Input: dimensioned drawing with shaded views. Units: mm. Origin: part minimum x, y, z. Give positions to 0.01 mm unless a question says otherwise; leave off trailing zeros. Order: outer loops, then holes, each group sorted by start corner. A loop starts at its lowest first (then second) coordinate and runs counter-clockwise, first axis right, second up. Notation, with made-up numbers: M -25,13.25 L 6,13.25 A18 cw 6,29.25 Z; hole C 34,22.25 d6. An arc over 180 degrees is marked long. Answer in a Markdown table with one row per item. Add a question column.
(1) Section query A-A, the plane x = 15. Return loops of the section in (y, z).
(2) Section query C-C, the plane y = 7. Return loops of the section in (x, z), plus the area to 3 significant figures.
(3) Material intervals for line 1 along Y through (x, z) = (28, 6); line 2 along Y through (x, z) = (32, 9.25); line 3 along X through (y, z) = (6.5, 8.75) (1 decimal), sorted ascending.
(4) Section query D-D, the plane y = 11. Return loops of the section in (x, z).
(5) Section query B-B, the plane z = 4. Return loops of the section in (x, y).
(6) Pin query (flat end, axial travel): P1, Ø1.5, axis at y = 10, z = 3.5, coming from the +X side; P2, Ø6, axis at x = 54, z = 1, coming from the -Y side. Return the tip coordinate at first contact, or that it passes through.
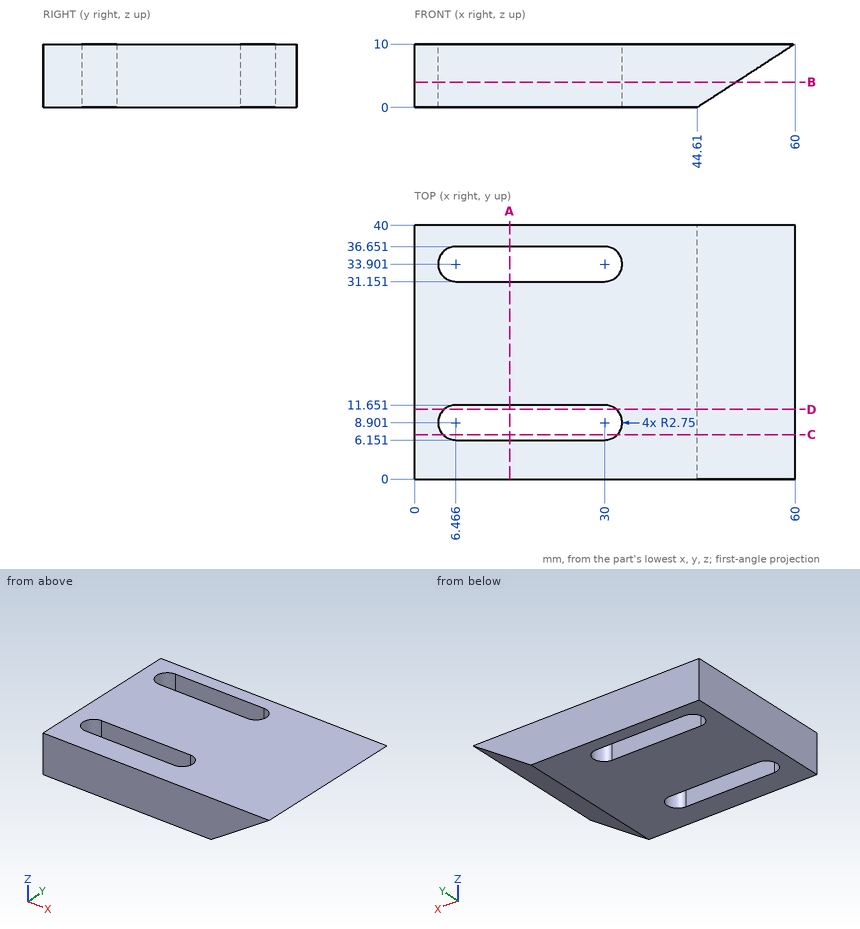
Values follow:
| question | item | result |
|---|---|---|
| 1 | outline | M 0,0 L 6.15,0 L 6.15,10 L 0,10 Z; M 11.65,0 L 31.15,0 L 31.15,10 L 11.65,10 Z; M 36.65,0 L 40,0 L 40,10 L 36.65,10 Z |
| 2 | outline | M 0,0 L 4.48,0 L 4.48,10 L 0,10 Z; M 31.99,0 L 44.61,0 L 60,10 L 31.99,10 Z |
| 2 | area | 248 mm² |
| 3 | line 1 | y = 0 to 6.15, 11.65 to 31.15, 36.65 to 40 |
| 3 | line 2 | y = 0 to 7.01, 10.79 to 32.01, 35.79 to 40 |
| 3 | line 3 | x = 0 to 5.1, 31.3 to 58.1 |
| 4 | outline | M 0,0 L 4.69,0 L 4.69,10 L 0,10 Z; M 31.78,0 L 44.61,0 L 60,10 L 31.78,10 Z |
| 5 | outline | M 0,0 L 50.77,0 L 50.77,40 L 0,40 Z; hole M 6.47,6.15 L 30,6.15 A2.75 ccw 30,11.65 L 6.47,11.65 A2.75 ccw Z; hole M 6.47,31.15 L 30,31.15 A2.75 ccw 30,36.65 L 6.47,36.65 A2.75 ccw Z |
| 6 | P1 | stops at x = 51.15 |
| 6 | P2 | passes through |
